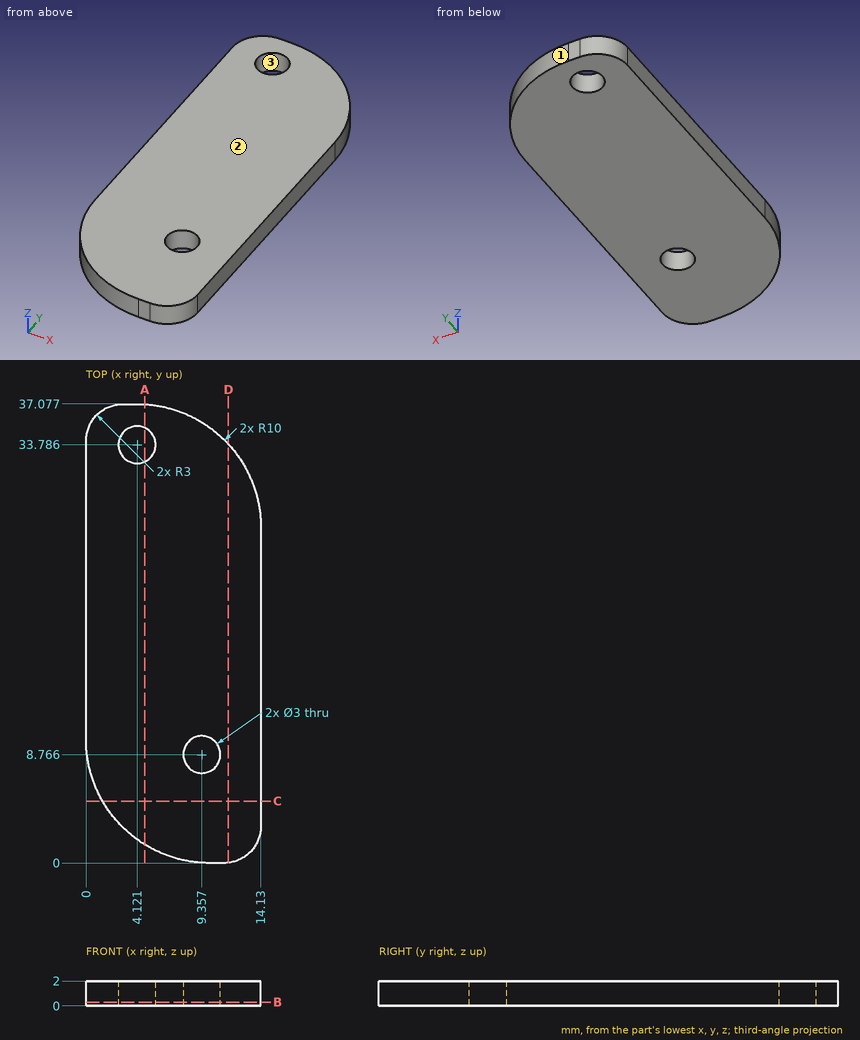
Geometry check sheet. Reference: drawing and pictorial views, mm from the part's lowest x, y, z. Give positions to 0.01 mm unless a question says otherwise; leave off trailing zeros. Order: outer loops, then holes, each group sorted by start corner. A loop starts at its lowest first (then second) coordinate and runs counter-clockwise, first axis right, second up. Notation, with made-up numbers: M -27.75,5.5 L -16.75,5.5 A31 cw -16.75,29.5 Z; hole C -2,-22.75 d9. An arc over 180 degrees is marked long. Answer in a Markdown table with one row per item. Add a question column.
Item 1: Gauge pin test, flat end, axial feed: pin 1 (2.5 mm diameter, centred on x = 4.12, y = 33.79, fed in from +Z). Record the tip position at first contact, or that the pin passes through.
Item 2: Section check A-A, the plane x = 4.75. Enter the section's corners in (y, z).
Item 3: Mould release check, pull along X, two halves, no side actions. Record for the marked faces 1, 2 and 3: released by +X, released by -X, zero draft, split by the parting line, or undercut.
Item 4: Section check D-D, the plane x = 11.5. Enter the section's corners in (y, z) (1 decimal).
Item 5: Scan lines: probe 1 along X at (y, z) = (8.5, 1.05); probe 2 along Y at (x, z) = (9.5, 1); probe 3 along X at (y, z) = (35, 0.85) (1 decimal). Record each from-to range of solid material in increasing order. Write a range as from..to.
Item 6: Section check C-C, the plane y = 5. Enter the section's corners in (x, z).
Item 7: Section check B-B, the plane z = 0.3. Enter the section's corners in (x, y) (1 decimal), and give its area (3 significant figures).
Filled sheet:
| question | item | result |
|---|---|---|
| 1 | pin 1 | passes through |
| 2 | outline | M 1.49,0 L 32.42,0 L 32.42,2 L 1.49,2 Z; M 35.15,0 L 37.06,0 L 37.06,2 L 35.15,2 Z |
| 3 | face 1 | released by +X |
| 3 | face 2 | zero draft |
| 3 | face 3 | undercut |
| 4 | outline | M 0,0 L 33.8,0 L 33.8,2 L 0,2 Z |
| 5 | probe 1 | x = 0.11..7.88, 10.83..14.13 |
| 5 | probe 2 | y = 0.01..7.27, 10.26..35.51 |
| 5 | probe 3 | x = 0.1..3.2, 5..10.2 |
| 6 | outline | M 1.34,0 L 14.13,0 L 14.13,2 L 1.34,2 Z |
| 7 | outline | M 0,10 A10 ccw 10,0 L 11.1,0 A3 ccw 14.1,3 L 14.1,27.1 A10 ccw 4.1,37.1 L 3,37.1 A3 ccw 0,34.1 Z; hole C 4.1,33.8 d3; hole C 9.4,8.8 d3 |
| 7 | area | 463 mm^2 |
